Study the drawing (mm; zero at the part's minimum x, y, z) and answer. A direction names the side the tool comes from. Coordinates: 2 decimals unless noted, no trailing zeros. Order: outer loops, then holes, each group sorted by start corner. A loop starts at its lowest first (then second) coordinate and runs counter-clockwise, first axis right, second up.
1. Flat-ended cylindrical pins translate along their axes: pin 1 Ø4 at (x, z) = (25.5, 10) entering from +Y; pin 2 Ø1.5 at (x, y) = (27, 3.5) entering from +Z; pin 3 Ø3 at (y, z) = (2, 20) entering from -X. Find the tip coordinate at first contact, or state that the pin passes through.
2. The part is cut by section D-D, the plane z = 4.75. Give the vertices of the cut face in (x, y), then the cut area to 4 significant figures.
3. Determine the mould class of the marked faces 5, 6, 7 and 8 for opening direction X: +X half, -X half, draft (parallel to the pull), parting line (faces both ways), or undercut.
4. The part is cut by section C-C, the plane x = 20. Give the vertices of the cut face in (y, z), then the cut area to 3 significant figures.
5. The part is cut by section B-B, the plane y = 0.45. Give the vertices of the cut face in (x, z), then the cut area to 3 significant figures.
6. A tool of negligible diameter and unlimited length cuts with its end or side. For the marked faces 1, 2, 3 and 4, from which of +Z, -Z, +X, -X, +Y, -Y can it reach the whole face along a straight path? Write none if from no direction.
7. The part is cut by section A-A, the plane y = 4.05. Give the vertices of the cut face in (x, z).
8. Find the intervals of material crossed by probe 1 along X at (y, z) = (2.1, 14.5); probe 2 along X at (y, z) = (3.4, 12); probe 3 along X at (y, z) = (3.6, 6.75), in increasing order.
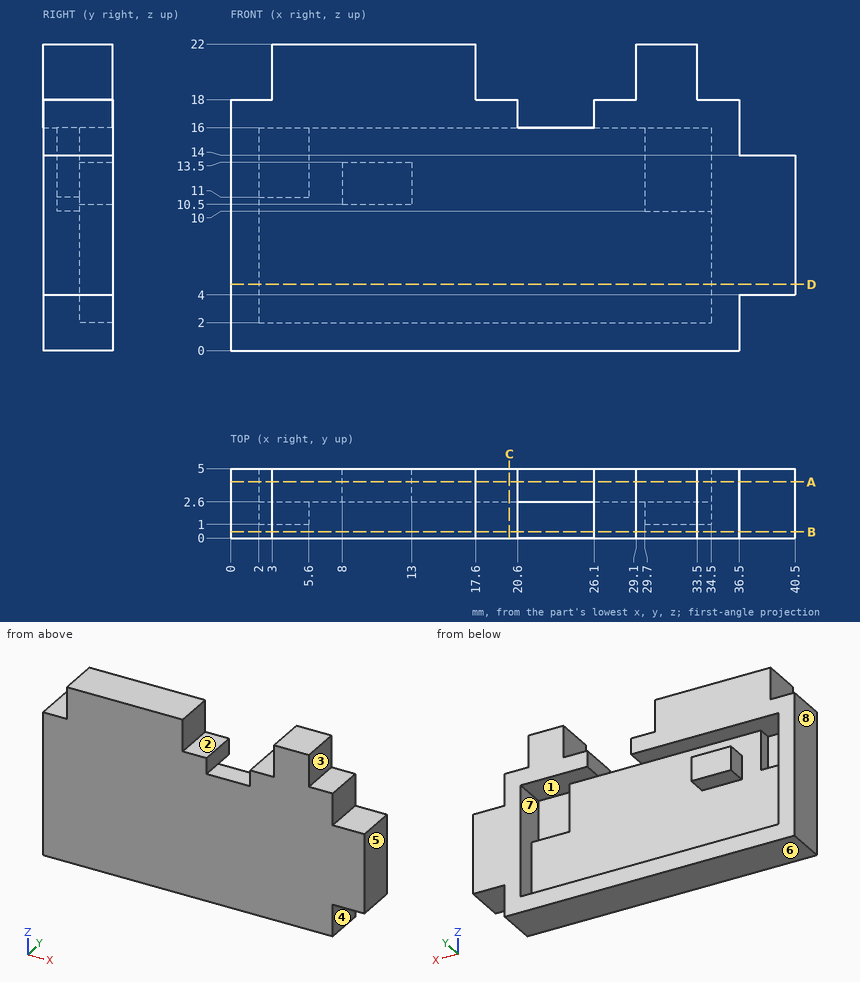
Geometry says:
1. pin 1: stops at y = 2.6
1. pin 2: stops at z = 18
1. pin 3: stops at x = 3
2. outline: (0, 0) - (40.5, 0) - (40.5, 5) - (34.5, 5) - (34.5, 2.6) - (2, 2.6) - (2, 5) - (0, 5) - close
2. area: 124.5 mm2
3. face 5: +X half
3. face 6: draft
3. face 7: undercut
3. face 8: -X half
4. outline: (0, 0) - (5, 0) - (5, 2) - (2.6, 2) - (2.6, 16) - (5, 16) - (5, 18) - (0, 18) - close
4. area: 56.4 mm2
5. outline: (0, 0) - (36.5, 0) - (36.5, 4) - (40.5, 4) - (40.5, 14) - (36.5, 14) - (36.5, 18) - (33.5, 18) - (33.5, 22) - (29.1, 22) - (29.1, 18) - (26.1, 18) - (26.1, 16) - (20.6, 16) - (20.6, 18) - (17.6, 18) - (17.6, 22) - (3, 22) - (3, 18) - (0, 18) - close
5. area: 762 mm2
6. face 1: +Y
6. face 2: +Z, +Y, -Y
6. face 3: +Z, +X, +Y, -Y
6. face 4: -Z, +X, +Y, -Y
7. outline: (0, 0) - (36.5, 0) - (36.5, 4) - (40.5, 4) - (40.5, 14) - (36.5, 14) - (36.5, 18) - (33.5, 18) - (33.5, 22) - (29.1, 22) - (29.1, 18) - (26.1, 18) - (26.1, 16) - (34.5, 16) - (34.5, 2) - (2, 2) - (2, 16) - (20.6, 16) - (20.6, 18) - (17.6, 18) - (17.6, 22) - (3, 22) - (3, 18) - (0, 18) - close; (8, 10.5) - (13, 10.5) - (13, 13.5) - (8, 13.5) - close
8. probe 1: x = 0 to 2, 5.6 to 29.7, 34.5 to 36.5
8. probe 2: x = 0 to 2, 8 to 13, 34.5 to 40.5
8. probe 3: x = 0 to 2, 34.5 to 40.5
